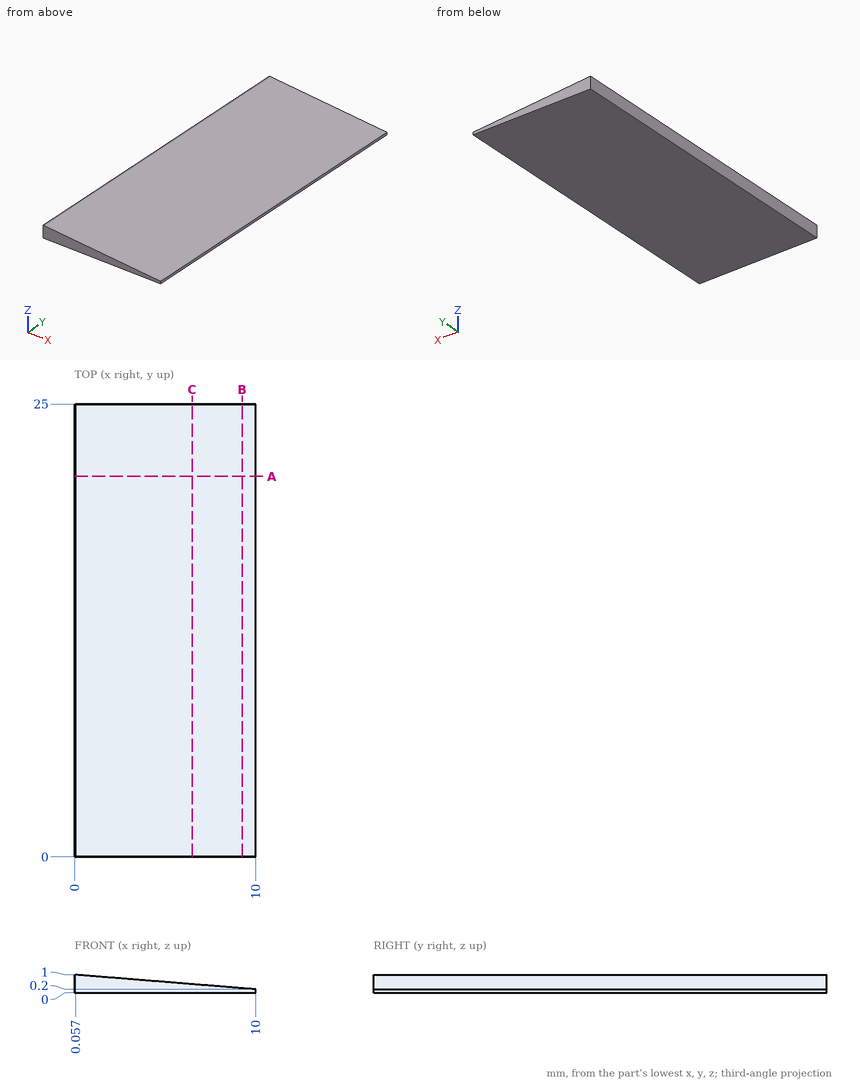
Part print with two shaded views. Sizes in mm from the minimum x, y, z corner. Round coordinates to 2 decimals unless told otherwise and drop trailing zeros. Order: outer loops, then holes, each group sorted by start corner. A loop starts at its lowest first (then second) coordinate and runs counter-clockwise, first axis right, second up. Notation, with made-up numbers: (86.5, 85.25) - (132.5, 85.25) arc R18 ccw to (132.5, 98.25) - close; hole circle Ø1 at (74.25, 60.25). An arc over 180 degrees is marked (long way). Answer in a Markdown table with one row per item. Add a question column.
(1) Probe L1, parallel to Z at x = 8, y = 9.5; L2, parallel to Z at x = 1.5, y = 17.5. List the from-to ranges inside material, lowest first. Write a range as [from, to].
(2) Band-saw the part on C-C on x = 6.5. List the corners of the cut face in (y, z), and give its area (3 significant figures).
(3) Drop flat-ended pins along their axis: pin 1 Ø2 at (x, y) = (3, 14) entering from -Z; pin 2 Ø1 at (x, y) = (6.5, 9.5) entering from +Z. Give the stop position or say it passes through.
(4) Band-saw the part on B-B on x = 9.25. List the corners of the cut face in (y, z).
(5) Band-saw the part on A-A on y = 21. List the corners of the cut face in (x, z).
Data:
| question | item | result |
|---|---|---|
| 1 | L1 | z = [0, 0.36] |
| 1 | L2 | z = [0, 0.88] |
| 2 | outline | (0, 0) - (25, 0) - (25, 0.48) - (0, 0.48) - close |
| 2 | area | 12.0 mm^2 |
| 3 | pin 1 | stops at z = 0 |
| 3 | pin 2 | stops at z = 0.52 |
| 4 | outline | (0, 0) - (25, 0) - (25, 0.26) - (0, 0.26) - close |
| 5 | outline | (0, 0) - (10, 0) - (10, 0.2) - (0.06, 1) - (0, 1) - close |
